```python
from build123d import *

# Parameters (mm, degrees)
SKETCH1_R           = 27.5
SKETCH1_R_2         = 6.65
BOSS_EXTRUDE1_DEPTH = 3
SKETCH3_R           = 1.6
CUT_EXTRUDE1_DEPTH  = 4


with BuildPart() as part:
    # Sketch1 → Boss-Extrude1 (new body)
    with BuildSketch(Plane(origin=(0, 0, 0), x_dir=(0, 0, -1), z_dir=(1, 0, 0))):
        Circle(SKETCH1_R)
        Circle(SKETCH1_R_2, mode=Mode.SUBTRACT)
    extrude(amount=BOSS_EXTRUDE1_DEPTH)

    # Sketch3 → Cut-Extrude1 (cut, through all)
    with BuildSketch(Plane(origin=(3, 0, 0), x_dir=(0, 0, -1), z_dir=(1, 0, 0))):
        with Locations((0, 17)):
            Circle(SKETCH3_R)
        with Locations((14.722431864, 8.5)):
            Circle(SKETCH3_R)
        with Locations((14.722431864, -8.5)):
            Circle(SKETCH3_R)
        with Locations((0, -17)):
            Circle(SKETCH3_R)
        with Locations((-14.722431864, -8.5)):
            Circle(SKETCH3_R)
        with Locations((-14.722431864, 8.5)):
            Circle(SKETCH3_R)
    extrude(amount=-CUT_EXTRUDE1_DEPTH, mode=Mode.SUBTRACT)


solid = part.part
```
Model file for the job. Use its own axes, mm. Round coordinates to 2 decimals unless told otherwise and drop trailing zeros. Write each loop counter-clockwise with the first axis right and the second up, starting at its lowest first coordinate (ties: lowest second). Pieces come first, ordered by that corner, then holes. Notation, with made-up numbers: (86, 50.5) - (135, 50.5) arc R23 cw to (135, 84.5) - close; hole circle Ø5 at (-29, 49.25). An arc over 180 degrees is marked (long way). Use CSV: the item, a comma, the result in double quotes. Start each with the question number.
Item 1: Drill centre lines: L1, parallel to Y at x = 2.7, z = 0; L2, parallel to Y at x = 2.6, z = 15.5; L3, parallel to Z at x = 2.6, y = -8. Where is each one in solid material? Low to high. Write a range as [from, to].
Item 2: Band-saw the part on A-A (x = 1.9). Write the cut outline in (y, z), and give its area (3 significant figures).
Item 3: Two-plate mould, pull along Y, no slides. Class faces 1 (the face through (3, -6, -6)), 2 (the face through (1.479, -26.846, 5.961)), 3 (the face through (1.521, -15.414, 0.208)): released by +Y, released by -Y, zero draft, split by the parting line, or undercut.
Item 4: Band-saw the part on D-D (y = -17). Write the cut outline in (x, z).
Item 5: Pin check, flat tip, straight feed: P1, Ø1, axis at x = 0.5, z = 20.5, coming from the -Y side. Stop position of the tip, or through.
Item 6: Band-saw the part on B-B (y = 0). Write the cut outline in (x, z).
Item 7: Band-saw the part on C-C (y = -8.5). Write the cut outline in (x, z).
Checked values:
1,L1,"y = [-27.5, -18.6], [-15.4, -6.65], [6.65, 15.4], [18.6, 27.5]"
1,L2,"y = [-22.72, -9.9], [-7.1, 7.1], [9.9, 22.72]"
1,L3,"z = [-26.31, -16.24], [-13.2, 13.2], [16.24, 26.31]"
2,outline,"circle Ø55 at (0, 0); hole circle Ø3.2 at (-17, 0); hole circle Ø3.2 at (-8.5, -14.72); hole circle Ø3.2 at (-8.5, 14.72); hole circle Ø13.3 at (0, 0); hole circle Ø3.2 at (8.5, -14.72); hole circle Ø3.2 at (8.5, 14.72); hole circle Ø3.2 at (17, 0)"
2,area,"2,190 mm²"
3,face 1,"zero draft"
3,face 2,"split by the parting line"
3,face 3,"undercut"
4,outline,"(0, -21.62) - (3, -21.62) - (3, -1.6) - (0, -1.6) - close; (0, 1.6) - (3, 1.6) - (3, 21.62) - (0, 21.62) - close"
5,P1,"stops at y = -18.87"
6,outline,"(0, -27.5) - (3, -27.5) - (3, -6.65) - (0, -6.65) - close; (0, 6.65) - (3, 6.65) - (3, 27.5) - (0, 27.5) - close"
7,outline,"(0, -26.15) - (3, -26.15) - (3, -16.32) - (0, -16.32) - close; (0, -13.12) - (3, -13.12) - (3, 13.12) - (0, 13.12) - close; (0, 16.32) - (3, 16.32) - (3, 26.15) - (0, 26.15) - close"
